```python
from build123d import *

# Parameters (mm, degrees)
SKETCH1_W           = 38
SKETCH1_H           = 38
SKETCH1_R           = 1
BOSS_EXTRUDE1_DEPTH = 4
BOSS_EXTRUDE2_START = 4
SKETCH2_R           = 7.3
BOSS_EXTRUDE2_DEPTH = 18


with BuildPart() as part:
    # Sketch1 → Boss-Extrude1 (new body)
    with BuildSketch(Plane.XY):
        Rectangle(SKETCH1_W, SKETCH1_H)
        with Locations((14, 14)):
            Circle(SKETCH1_R, mode=Mode.SUBTRACT)
        with Locations((17, 17)):
            Circle(SKETCH1_R, mode=Mode.SUBTRACT)
        with Locations(Location((14, -14, 0), (0, 0, 180))):
            Circle(SKETCH1_R, mode=Mode.SUBTRACT)
        with Locations(Location((17, -17, 0), (0, 0, 180))):
            Circle(SKETCH1_R, mode=Mode.SUBTRACT)
        with Locations((-14, -14)):
            Circle(SKETCH1_R, mode=Mode.SUBTRACT)
        with Locations((-17, -17)):
            Circle(SKETCH1_R, mode=Mode.SUBTRACT)
        with Locations(Location((-17, 17, 0), (0, 0, 180))):
            Circle(SKETCH1_R, mode=Mode.SUBTRACT)
        with Locations(Location((-14, 14, 0), (0, 0, 180))):
            Circle(SKETCH1_R, mode=Mode.SUBTRACT)
    extrude(amount=BOSS_EXTRUDE1_DEPTH)

    # Sketch2 → Boss-Extrude2 (add)
    with BuildSketch(Plane.XY.offset(BOSS_EXTRUDE2_START)):
        with Locations(Location((0, 0, 0), (0, 0, 180))):
            Circle(SKETCH2_R)
    extrude(amount=BOSS_EXTRUDE2_DEPTH)


solid = part.part
```
Could you check a few things on this model? Use its own coordinates, in mm. A direction names the side the tool comes from. Coordinates: 2 decimals unless noted, no trailing zeros. Order: outer loops, then holes, each group sorted by start corner. A loop starts at its lowest first (then second) coordinate and runs counter-clockwise, first axis right, second up. Notation, with made-up numbers: M -25,45 L -16,45 A22 ccw -16,51 Z; hole C -39,53.25 d8. An arc over 180 degrees is marked long. Use a Markdown table: item, result. Add a question column.
Q1. If I drill on L1, parallel to Y at x = 17, z = 3.1; L2, parallel to Y at x = -14, z = 3.15; L3, parallel to Z at x = 11.5, y = -5, over which ranges is the centre line in solid material (lowest first)?
Q2. We'd pull the mould along X, two halves only. Please class faces 1 (the cylindrical face through (17, 16, 2)), 2 (the flat face through (-19, 0, 2)), 3 (the cylindrical face through (-14, 15, 2)), 4 (the flat face through (0, 19, 2)): pulls with the +X half, pulls with the -X half, needs draft (parallel to the pull), parting line crosses it, or undercut.
Q3. I want a section at D-D on y = 0. List the corners of the cut face in (x, z) for me.
Q4. Which directions (+Z, -Z, +X, -X, +Y, -Y) give clear straight access to the entire face, cutting with the end or side of a thin tool? Please do faces 5 (the cylindrical face through (-6.963, -2.193, 12.874)), 6 (the cylindrical face through (-17, 18, 2)).
Q5. I want a section at C-C on z = 1.5. Give the number of separate pieces and of enclosed holes in the cut face, then the cut area to 3 significant figures.
Q6. I'm going to push flat-ended pins straight in: pin 1 (1.6 mm diameter, centred on x = -17, y = 17, fed in from -Z); pin 2 (3 mm diameter, centred on x = 14, y = -14, fed in from +Z); pin 3 (12 mm diameter, centred on y = -10, z = 14, fed in from -X); pin 4 (8 mm diameter, centred on y = -7.5, z = 10.5, fed in from -X). Where does each tip first touch, or does it pass through?
Q7. I want a section at A-A on y = 17. List the corners of the cut face in (x, z) for me, then the cut area to 3 significant figures.
Q8. I want a section at B-B on x = -14. List the corners of the cut face in (y, z) for me, then the cut area to 3 significant figures.
Checked values:
| question | item | result |
|---|---|---|
| 1 | L1 | -19 to -18, -16 to 16, 18 to 19 |
| 1 | L2 | -19 to -15, -13 to 13, 15 to 19 |
| 1 | L3 | 0 to 4 |
| 2 | face 1 | undercut |
| 2 | face 2 | pulls with the -X half |
| 2 | face 3 | undercut |
| 2 | face 4 | needs draft |
| 3 | outline | M -19,0 L 19,0 L 19,4 L 7.3,4 L 7.3,22 L -7.3,22 L -7.3,4 L -19,4 Z |
| 4 | face 5 | +Z |
| 4 | face 6 | +Z, -Z |
| 5 | separate pieces | 1 |
| 5 | enclosed holes | 8 |
| 5 | area | 1,420 mm² |
| 6 | pin 1 | through |
| 6 | pin 2 | z = 4 |
| 6 | pin 3 | x = -6.11 |
| 6 | pin 4 | x = -6.41 |
| 7 | outline | M -19,0 L -18,0 L -18,4 L -19,4 Z; M -16,0 L 16,0 L 16,4 L -16,4 Z; M 18,0 L 19,0 L 19,4 L 18,4 Z |
| 7 | area | 136 mm² |
| 8 | outline | M -19,0 L -15,0 L -15,4 L -19,4 Z; M -13,0 L 13,0 L 13,4 L -13,4 Z; M 15,0 L 19,0 L 19,4 L 15,4 Z |
| 8 | area | 136 mm² |
